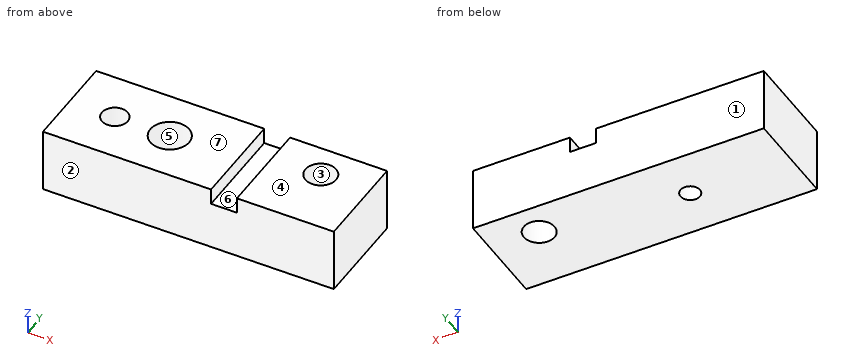
```python
from build123d import *

# Parameters (mm, degrees)
SKETCH_1_W          = 90
SKETCH_1_H          = 30
EXTRUDE_1_DEPTH     = 20
SKETCH_2_W          = 8
SKETCH_2_H          = 30
CUT_EXTRUDE_1_DEPTH = 5
SKETCH_8_R          = 4.75
CUT_EXTRUDE_4_DEPTH = 97.953597148


with BuildPart() as part:
    # Эскиз1 → Бобышка-Вытянуть1 (new body)
    with BuildSketch(Plane.XY):
        with Locations((45, 15)):
            Rectangle(SKETCH_1_W, SKETCH_1_H)
    extrude(amount=-EXTRUDE_1_DEPTH)

    # Эскиз2 → Вырез-Вытянуть1 (cut)
    with BuildSketch(Plane.XY):
        with Locations((56, 15)):
            Rectangle(SKETCH_2_W, SKETCH_2_H)
    extrude(amount=-CUT_EXTRUDE_1_DEPTH, mode=Mode.SUBTRACT)

    # Эскиз8 → Вырез-Вытянуть4 (cut, through all)
    with BuildSketch(Plane.XY):
        with Locations((75, 20)):
            Circle(SKETCH_8_R)
    extrude(amount=-CUT_EXTRUDE_4_DEPTH, mode=Mode.SUBTRACT)

    # Эскиз5 → Вырез-Повернуть1 (revolve, cut)
    with BuildSketch(Plane(origin=(0, 15, 0), x_dir=(1, 0, 0), z_dir=(0, 1, 0))):
        Polygon((31, 0), (37, 0), (37, 12), (34, 12), (34, 20), (31, 20), align=None)
    revolve(axis=Axis((31, 15, 0), (0, 0, -1)), mode=Mode.SUBTRACT)

    # Эскиз6 → Вырез-Повернуть2 (revolve, cut)
    with BuildSketch(Plane(origin=(0, 15, 0), x_dir=(1, 0, 0), z_dir=(0, 1, 0))):
        Polygon((14, 0), (18, 0), (18, 10), (14, 12.309401077), align=None)
    revolve(axis=Axis((14, 15, 0), (0, 0, -1)), mode=Mode.SUBTRACT)


solid = part.part
```
Geometry: final body of the model. Coordinates: model frame, mm. Face numbers are marked on the shaded views. A direction names the side the tool comes from. Coordinates: 2 decimals unless noted, no trailing zeros. Order: outer loops, then holes, each group sorted by start corner. A loop starts at its lowest first (then second) coordinate and runs counter-clockwise, first axis right, second up. Notation, with made-up numbers: M 49,17.25 L 53,17.25 A27 ccw 53,46.25 Z; hole C -27.5,19 d3. An arc over 180 degrees is marked long. Answer as CSV lines item,"result".
Q1. Section C-C on y = 20. Return the cut outline in (x, z), and give its area (3 significant figures).
Answers:
outline,"M 0,-20 L 70.25,-20 L 70.25,0 L 60,0 L 60,-5 L 52,-5 L 52,0 L 34.32,0 L 34.32,-12 L 27.68,-12 L 27.68,0 L 0,0 Z; M 79.75,-20 L 90,-20 L 90,0 L 79.75,0 Z"
area,"1,490 mm^2"
Q2. Draft query along Y for the marked faces 1, 2, 3 and 4. Return one class per face: pulls with the +Y half, pulls with the -Y half, needs draft (parallel to the pull), parting line crosses it, or undercut.
Answers:
face 1,"pulls with the +Y half"
face 2,"pulls with the -Y half"
face 3,"undercut"
face 4,"needs draft"
Q3. Set-up query: the marked faces 5, 6 and 7. Return all of +Z, -Z, +X, -X, +Y, -Y with unobstructed straight access to the full face (end or side cutting, diameter ignored); none if empty.
Answers:
face 5,"+Z"
face 6,"+Z, +Y, -Y"
face 7,"+Z, +X, -X, +Y, -Y"
Q4. Section A-A on x = 31. Return the cut outline in (y, z).
Answers:
outline,"M 0,-20 L 12,-20 L 12,-12 L 9,-12 L 9,0 L 0,0 Z; M 18,-20 L 30,-20 L 30,0 L 21,0 L 21,-12 L 18,-12 Z"
Q5. Section D-D on y = 3.5. Return the cut outline in (x, z).
Answers:
outline,"M 0,-20 L 90,-20 L 90,0 L 60,0 L 60,-5 L 52,-5 L 52,0 L 0,0 Z"
Q6. First-contact query: P1, Ø3.5, axis at x = 30, y = 15.5, coming from the +Z side; P2, Ø2.5, axis at x = 54.5, y = 15.5, coming from the +Z side; P3, Ø9.5, axis at x = 31, y = 15, coming from the +Z side. Flat tips, straight axial feed; report the tip coordinate or a pass-through.
Answers:
P1,"passes through"
P2,"stops at z = -5"
P3,"stops at z = -12"
Q7. Section B-B on z = -7.75. Return the cut outline in (x, y), and give its area (3 significant figures).
Answers:
outline,"M 0,0 L 90,0 L 90,30 L 0,30 Z; hole C 14,15 d8; hole C 31,15 d12; hole C 75,20 d9.5"
area,"2,470 mm^2"
Q8. Line query: probe 1 along X at (y, z) = (15, -5.25); probe 2 along X at (y, z) = (15, -1.75); probe 3 along X at (y, z) = (28.75, -4). Output: solid intervals per line, ascending. Write a range as [from, to].
Answers:
probe 1,"x = [0, 10], [18, 25], [37, 90]"
probe 2,"x = [0, 10], [18, 25], [37, 52], [60, 90]"
probe 3,"x = [0, 52], [60, 90]"
